The listing builds one solid part. Answer for the finished solid, in the listing's coordinates (mm). A direction names the side the tool comes from. Coordinates: 2 decimals unless noted, no trailing zeros. Order: outer loops, then holes, each group sorted by start corner. A loop starts at its lowest first (then second) coordinate and runs counter-clockwise, first axis right, second up. Notation, with made-up numbers: (-1.5, 26) -> (35.5, 26) arc R13 cw to (35.5, 39) -> close; hole circle Ø8 at (58, 9.5). An arc over 180 degrees is marked (long way). Return JSON: item names as keys, results as strings.
```python
from build123d import *

# Parameters (mm, degrees)
SKETCH1_R            = 10.000000000000009
BOSS_EXTRUDE1_DEPTH  = 27
CUT_EXTRUDE3_DEPTH   = 157.18313390219527
SKETCH2_R            = 1.5000000000000042
CUT_EXTRUDE4_DEPTH   = 157.18313390219527
LPATTERN1_COUNT      = 4
LPATTERN1_PITCH      = 35
LPATTERN1_COUNT_DIR2 = 2
LPATTERN1_PITCH_DIR2 = 55
LPATTERN2_COUNT      = 2
LPATTERN2_PITCH      = 20
FILLET1_R            = 5
FILLET2_R            = 5
BOSS_EXTRUDE2_DEPTH  = 104
FILLET3_R            = 5
FILLET4_R            = 5
SKETCH13_R           = 1.4999999999999973
SKETCH13_R_2         = 1.4999999999999971
CUT_EXTRUDE8_DEPTH   = 163.89624264715565


with BuildPart() as part:
    # Sketch1 → Boss-Extrude1 (new body)
    # profile 1 of 2: a face of its own
    with BuildSketch(Plane.XY):
        with BuildLine():
            Line((128.8099999999999, 22), (63.80000000000001, 22))
            Line((63.800000000000026, 22), (63.800000000000026, -22.136002859999998))
            Line((63.80000000000001, -22.136002859999998), (128.8099999999999, -22.136002859999998))
            ThreePointArc((128.8099999999999, -22.136002859999998), (150.8780014299999, -0.06800142999999757), (128.8099999999999, 22))
        make_face()
        with Locations((128.81, 0)):
            Circle(SKETCH1_R, mode=Mode.SUBTRACT)
    # profile 2 of 2: a face of its own
    with BuildSketch(Plane.XY):
        with BuildLine():
            Line((-58.799999999999976, 29.999999999999993), (58.80000000000002, 29.999999999999993))
            ThreePointArc((58.80000000000002, 29.999999999999993), (62.33553390593276, 28.535533905932734), (63.800000000000026, 24.999999999999993))
            Line((63.800000000000026, 24.999999999999993), (63.800000000000026, -25))
            ThreePointArc((63.800000000000026, -25), (62.33553390593277, -28.53553390593274), (58.80000000000003, -30.000000000000004))
            Line((58.80000000000003, -30.000000000000004), (-58.79999999999999, -30.000000000000004))
            ThreePointArc((-58.79999999999999, -30.000000000000004), (-62.33553390593272, -28.535533905932734), (-63.79999999999998, -25))
            Line((-63.79999999999998, -25), (-63.79999999999998, 24.999999999999993))
            ThreePointArc((-63.79999999999998, 24.999999999999993), (-62.335533905932714, 28.53553390593273), (-58.799999999999976, 29.999999999999993))
        make_face()
    extrude(amount=BOSS_EXTRUDE1_DEPTH)

    # Sketch4 → Cut-Extrude3 (cut, through all)
    with BuildSketch(Plane.XY.offset(27)):
        with BuildLine():
            Line((128.8099999999999, 16.999999999999996), (58.800000000000026, 16.999999999999996))
            Line((58.800000000000026, 16.999999999999996), (58.800000000000026, 24.99999999999999))
            Line((58.800000000000026, 24.99999999999999), (-58.79999999999998, 24.99999999999999))
            Line((-58.79999999999998, 24.99999999999999), (-58.79999999999998, -25))
            Line((-58.79999999999998, -25), (58.800000000000026, -25))
            Line((58.800000000000026, -25), (58.800000000000026, -17.136002859999994))
            Line((58.800000000000026, -17.136002859999994), (128.8099999999999, -17.136002859999994))
            ThreePointArc((128.8099999999999, -17.136002859999994), (145.87800142999987, -0.06800142999999897), (128.8099999999999, 16.999999999999996))
        make_face()
    extrude(amount=-CUT_EXTRUDE3_DEPTH, mode=Mode.SUBTRACT)

    # Sketch2 → Cut-Extrude4 (cut, through all)
    with BuildSketch(Plane.XY.offset(27)):
        with Locations((-51.19999999999998, 27.49999999999999)):
            Circle(SKETCH2_R)
        with Locations((-61.29999999999998, 9.999999999999991)):
            Circle(SKETCH2_R)
    cut_extrude4 = extrude(amount=-CUT_EXTRUDE4_DEPTH, mode=Mode.SUBTRACT)

    # LPattern1: Cut-Extrude4 4 × 2
    with Locations(*[(i * LPATTERN1_PITCH, -j * LPATTERN1_PITCH_DIR2, 0) for i in range(LPATTERN1_COUNT) for j in range(LPATTERN1_COUNT_DIR2) if (i, j) != (0, 0)]):
        add(cut_extrude4, mode=Mode.SUBTRACT)

    # LPattern2: Cut-Extrude4 ×2
    with Locations(*[(0, -i * LPATTERN2_PITCH, 0) for i in range(1, LPATTERN2_COUNT)]):
        add(cut_extrude4, mode=Mode.SUBTRACT)

    # Fillet1
    fillet1_edges = [part.edges().sort_by_distance(p)[0] for p in [
        (58.800000000000026, -17.136002859999994, 13.5),
        (58.800000000000026, 16.999999999999996, 13.5),
    ]]
    fillet(fillet1_edges, radius=FILLET1_R)

    # Fillet2
    fillet2_edges = [part.edges().sort_by_distance(p)[0] for p in [
        (-58.79999999999998, -25, 13.5),
        (-58.79999999999998, 24.99999999999999, 13.5),
    ]]
    fillet(fillet2_edges, radius=FILLET2_R)

    # Sketch6 → Boss-Extrude2 (add)
    with BuildSketch(Plane.ZY.offset(58.79999999999998)):
        with BuildLine():
            Line((27, 29.999999999999993), (27, 39.99999999999999))
            ThreePointArc((27, 39.99999999999999), (9.251807345621204, 53.9041792903447), (0, 33.34381438418348))
            Line((0, 33.34381438418348), (2.6562431277765906, 34.738221945171176))
            ThreePointArc((2.6562431277765906, 34.738221945171176), (9.969884854205839, 50.99138601040448), (24, 39.99999999999999))
            Line((24, 39.99999999999999), (24, 29.999999999999993))
            Line((24, 29.999999999999993), (27, 29.999999999999993))
        make_face()
    extrude(amount=-BOSS_EXTRUDE2_DEPTH)

    # Fillet3
    # the kernel refuses this fillet: 5 mm, written as the material it takes off along each edge
    with BuildSketch(Plane(origin=(-58.79999999999998, 18.543560762610387, 27), x_dir=(1, 0, 0), z_dir=(0, 1, 0))) as fillet3_piece_1_section:
        with BuildLine():
            CenterArc((4.5825756949558425, 5), FILLET3_R, 203.57817847820183, 66.42182152179817)
            Line((0, 3), (0, 0))
            Line((0, 0), (4.5825756949558425, 0))
        make_face()
    fillet3_piece_1 = extrude(amount=21.456439237389606, mode=Mode.PRIVATE)
    fillet3_piece_1 = fillet3_piece_1 - Plane(origin=(-58.79999999999997, 24.99999999999998, 26.19166673293572), x_dir=(-1, 2.84e-15, 0), z_dir=(0, 0, -1)) * Cylinder(5.000000000000014, 62, mode=Mode.PRIVATE)
    add(fillet3_piece_1, mode=Mode.SUBTRACT)
    with BuildSketch(Plane(origin=(-58.79999999999998, 39.999999999999986, 12.679540611996243), x_dir=(0, 5e-16, 1), z_dir=(0, -1, 5e-16))) as fillet3_piece_2_section:
        with BuildLine():
            CenterArc((9.320459388003757, -4.5825756949558425), FILLET3_R, 0, 66.42182152179822)
            Line((14.320459388003757, -4.5825756949558425), (14.320459388003757, 0))
            Line((14.320459388003757, 0), (11.320459388003753, 0))
        make_face()
    fillet3_piece_2 = revolve(axis=Axis((-58.79999999999998, 39.999999999999986, 12.679540611996243), (-1, 0, 0)), revolution_arc=253.63253481622772, mode=Mode.PRIVATE)
    fillet3_piece_2 = split(fillet3_piece_2, bisect_by=Plane(origin=(-58.68295720401122, 29.999999999999993, 23.934406963840928), z_dir=(0, 1, 0)), keep=Keep.TOP, mode=Mode.PRIVATE)
    add(fillet3_piece_2, mode=Mode.SUBTRACT)

    # Fillet4
    # the kernel refuses this fillet: 5 mm, written as the material it takes off along each edge
    with BuildSketch(Plane(origin=(45.20000000000002, 29.999999999999993, 27), x_dir=(-1, 0, 0), z_dir=(0, 1, 0))) as fillet4_piece_1:
        with BuildLine():
            CenterArc((4.5825756949558425, -5), FILLET4_R, 90, 66.42182152179817)
            Line((0, -3), (0, 0))
            Line((0, 0), (4.5825756949558425, 0))
        make_face()
    extrude(amount=10, mode=Mode.SUBTRACT)
    with BuildSketch(Plane(origin=(45.20000000000002, 39.999999999999986, 12.679540611996243), x_dir=(0, 5e-16, 1), z_dir=(0, -1, 5e-16))) as fillet4_piece_2_section:
        with BuildLine():
            CenterArc((9.320459388003757, 4.582575694955835), FILLET4_R, 293.57817847820183, 66.42182152179817)
            Line((11.320459388003757, -7.11e-15), (14.320459388003757, 0))
            Line((14.320459388003757, 0), (14.320459388003757, 4.582575694955835))
        make_face()
    fillet4_piece_2 = revolve(axis=Axis((45.20000000000002, 39.999999999999986, 12.679540611996243), (-1, 0, 0)), revolution_arc=253.63253481622772, mode=Mode.PRIVATE)
    fillet4_piece_2 = split(fillet4_piece_2, bisect_by=Plane(origin=(43.36151431814506, 29.999999999999993, 25.79888399879933), z_dir=(0, 1, 0)), keep=Keep.TOP, mode=Mode.PRIVATE)
    add(fillet4_piece_2, mode=Mode.SUBTRACT)

    # Sketch13 → Cut-Extrude8 (cut, through all)
    with BuildSketch(Plane.XY.offset(27)):
        with Locations((68.8099999999999, 19.5)):
            Circle(SKETCH13_R)
        with Locations((88.8099999999999, 19.5)):
            Circle(SKETCH13_R)
        with Locations((108.8099999999999, 19.5)):
            Circle(SKETCH13_R)
        with Locations((128.8099999999999, 19.5)):
            Circle(SKETCH13_R)
        with Locations((88.8100000000003, -19.64)):
            Circle(SKETCH13_R)
        with Locations((108.81000000000031, -19.64)):
            Circle(SKETCH13_R)
        with Locations((128.81000000000031, -19.64)):
            Circle(SKETCH13_R)
        with Locations((68.8100000000003, -19.64)):
            Circle(SKETCH13_R)
        with Locations((148.3099999999999, 0)):
            Circle(SKETCH13_R_2)
    extrude(amount=-CUT_EXTRUDE8_DEPTH, mode=Mode.SUBTRACT)


solid = part.part
```
Item 1: Which of the six approach directions +Z, -Z, +X, -X, +Y, -Y give full straight-line access (tool end or side, diameter ignored) to faces 1 (the cylindrical face through (60.304, -18.562, 13.311)), 2 (the flat face through (36, -27, 0)), 3 (the flat face through (-8, 35, 24))?
Answer list:
{"face 1": "+Z, -Z", "face 2": "-Z, +X, -X, -Y", "face 3": "+X, -X"}
Item 2: The part is cut by section B-B on y = -4. Determine the outline of the cut face in (x, z).
Answer list:
{"outline": "(-63.8, 0) -> (-58.8, 0) -> (-58.8, 27) -> (-63.8, 27) -> close; (145.42, 0) -> (150.52, 0) -> (150.52, 27) -> (145.42, 27) -> close"}
Item 3: The part is cut by section C-C on z = 20.5. Count the separate pieces of the cut face and the enclosed holes in it, plus the area to 3 significant figures.
Answer list:
{"separate pieces": "2", "enclosed holes": "20", "area": "2,790 mm2"}
Item 4: Flat-ended cylindrical pins translate along their axes: pin 1 (5 mm diameter, centred on y = -13, z = 2, fed in from +X); pin 2 (13.5 mm diameter, centred on y = 2, z = 8, fed in from +X); pin 3 (18 mm diameter, centred on x = 68, y = -9, fed in from -Z). Find the tip coordinate at first contact, or state that the pin passes through.
Answer list:
{"pin 1": "x = 148.26", "pin 2": "x = 150.88", "pin 3": "z = 0"}
Item 5: Find the intervals of material crossed by probe 1 along Y at (x, z) = (108.81, 14.5); probe 2 along Y at (x, z) = (-4.5, 17); probe 3 along X at (y, z) = (27.5, 6.75), in increasing order.
Answer list:
{"probe 1": "-22.14 to -21.14, -18.14 to -17.14, 17 to 18, 21 to 22", "probe 2": "-30 to -25, 25 to 30, 50.46 to 53.65", "probe 3": "-63.13 to -52.7, -49.7 to -17.7, -14.7 to 17.3, 20.3 to 52.3, 55.3 to 63.13"}
Item 6: The part is cut by section A-A on x = 97.5. Determine the outline of the cut face in (y, z), plus the area to 3 significant figures.
Answer list:
{"outline": "(-22.14, 0) -> (-17.14, 0) -> (-17.14, 27) -> (-22.14, 27) -> close; (17, 0) -> (22, 0) -> (22, 27) -> (17, 27) -> close", "area": "270 mm2"}
Item 7: The part is cut by section D-D on x = 24. Determine the outline of the cut face in (y, z).
Answer list:
{"outline": "(-30, 0) -> (-25, 0) -> (-25, 27) -> (-30, 27) -> close; (25, 0) -> (30, 0) -> (30, 24) -> (40, 24) arc R11.32 cw (long way) to (34.74, 2.66) -> (33.34, 0) arc R14.32 ccw (long way) to (40, 27) -> (25, 27) -> close"}
Item 8: Determine the mould class of faces 4 (the flat face through (-1, 30, 14)), 5 (the flat face through (96, -17.136, 14)), 6 (the flat face through (97, 17, 14)), 7 (the cylindrical face through (-62.3, -28.57, 13.31)) for opening direction X: pulls with the +X half, pulls with the -X half, needs draft (parallel to the pull), parting line crosses it, or undercut.
Answer list:
{"face 4": "needs draft", "face 5": "undercut", "face 6": "undercut", "face 7": "pulls with the -X half"}
